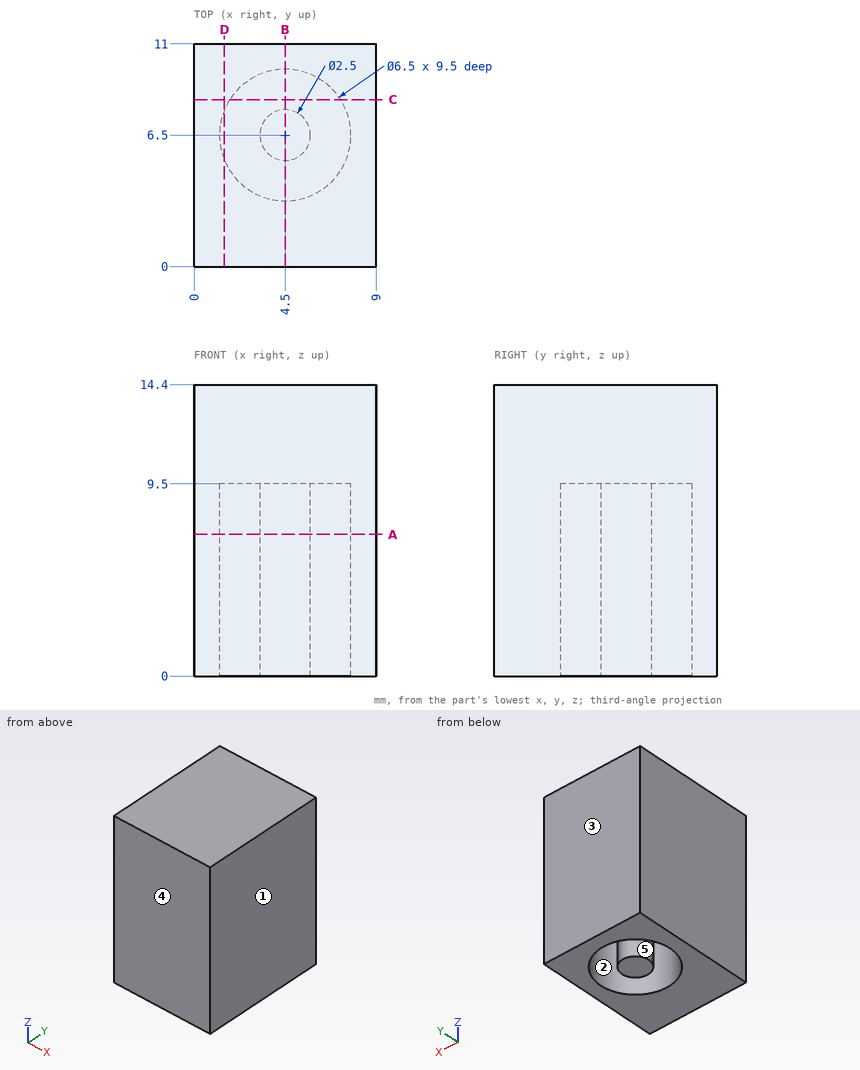
Here's the drawing with two shaded views (mm, measured from the low corner). I have some questions. A direction names the side the tool comes from. Give positions to 0.01 mm unless a question says otherwise; leave off trailing zeros. Write each loop counter-clockwise with the first axis right and the second up, starting at its lowest first coordinate (ties: lowest second). Pieces come first, ordered by that corner, then holes. Notation, with made-up numbers: (70, 31) -> (80, 31) arc R29 ccw to (80, 53) -> close; hole circle Ø8 at (17.25, 3). An arc over 180 degrees is marked (long way). One line per item, written item: value.
Q1. Imagine slicing it at A-A on z = 7. Please give me the cut outline in (x, y), and give its area (3 significant figures).
Results found:
outline: (0, 0) -> (9, 0) -> (9, 11) -> (0, 11) -> close; circle Ø2.5 at (4.5, 6.5); hole circle Ø6.5 at (4.5, 6.5)
area: 70.7 mm^2
Q2. Which directions (+Z, -Z, +X, -X, +Y, -Y) give clear straight access to the entire face, cutting with the end or side of a thin tool? Please do the marked faces 4 and 5.
Results found:
face 4: +Z, -Z, +X, -X, -Y
face 5: -Z
Q3. Imagine slicing it at C-C on y = 8.25. Please give me the cut outline in (x, z).
Results found:
outline: (0, 0) -> (1.76, 0) -> (1.76, 9.5) -> (7.24, 9.5) -> (7.24, 0) -> (9, 0) -> (9, 14.4) -> (0, 14.4) -> close
Q4. Imagine slicing it at D-D on x = 1.5. Please give me the cut outline in (y, z), and give its area (3 significant figures).
Results found:
outline: (0, 0) -> (5.25, 0) -> (5.25, 9.5) -> (7.75, 9.5) -> (7.75, 0) -> (11, 0) -> (11, 14.4) -> (0, 14.4) -> close
area: 135 mm^2
Q5. For P1, Ø2, axis at x = 3.5, y = 5, coming from the -Z side, with a flat end and sliding along its axis, tell me the tip position at first contact or that it passes through.
Results found:
P1: stops at z = 0
Q6. Imagine slicing it at B-B on x = 4.5. Please give me the cut outline in (y, z).
Results found:
outline: (0, 0) -> (3.25, 0) -> (3.25, 9.5) -> (5.25, 9.5) -> (5.25, 0) -> (7.75, 0) -> (7.75, 9.5) -> (9.75, 9.5) -> (9.75, 0) -> (11, 0) -> (11, 14.4) -> (0, 14.4) -> close
Q7. We'd pull the mould along X, two halves only. Please class the marked faces 1, 2 and 3: +X half, -X half, draft (parallel to the pull), parting line (faces both ways), or undercut.
Results found:
face 1: +X half
face 2: undercut
face 3: draft
Q8. Please list where these lines run through material, in increasing order: line 1 (Y direction, x = 4.5, z = 3.25); line 2 (Y direction, x = 5.5, z = 7.25); line 3 (Z direction, x = 3.5, y = 8.5). Write a range as [from, to].
Results found:
line 1: y = [0, 3.25], [5.25, 7.75], [9.75, 11]
line 2: y = [0, 3.41], [5.75, 7.25], [9.59, 11]
line 3: z = [9.5, 14.4]
